from build123d import *

# Parameters (mm, degrees)
SKETCH1_W           = 30
SKETCH1_H           = 100
BOSS_EXTRUDE1_DEPTH = 10
SKETCH2_R           = 5
CUT_EXTRUDE1_DEPTH  = 10
SKETCH3_W           = 100
SKETCH3_H           = 40
BOSS_EXTRUDE2_DEPTH = 50
FILLET1_R           = 10


with BuildPart() as part:
    # Sketch1 → Boss-Extrude1 (new body)
    with BuildSketch(Plane(origin=(0, 0, 0), x_dir=(1, 0, 0), z_dir=(0, 1, 0))):
        Rectangle(SKETCH1_W, SKETCH1_H)
    extrude(amount=BOSS_EXTRUDE1_DEPTH)

    # Sketch2 → Cut-Extrude1 (cut)
    with BuildSketch(Plane(origin=(0, 10, 0), x_dir=(1, 0, 0), z_dir=(0, 1, 0))):
        with Locations(Location((0, -40, 0), (0, 0, 270))):
            Circle(SKETCH2_R)
    extrude(amount=-CUT_EXTRUDE1_DEPTH, mode=Mode.SUBTRACT)

    # Sketch3 → Boss-Extrude2 (add)
    with BuildSketch(Plane(origin=(0, 0, -50), x_dir=(-1, 0, 0), z_dir=(0, 0, -1))):
        with Locations((0, 5)):
            Rectangle(SKETCH3_W, SKETCH3_H)
    extrude(amount=-BOSS_EXTRUDE2_DEPTH)

    # Fillet1
    fillet1_edges = [part.edges().sort_by_distance(p)[0] for p in [
        (15, 5, 50),
        (-15, 5, 50),
    ]]
    fillet(fillet1_edges, radius=FILLET1_R)


solid = part.part
Model file for the job. Use its own axes, mm. A direction names the side the tool comes from. Give positions to 0.01 mm unless a question says otherwise; leave off trailing zeros. Loops run counter-clockwise (first coordinate to the right, second up) from the corner with the lowest first, then second, coordinate; pieces in that order, holes last.
Item 1: Drill centre lines: line 1 along X through (y, z) = (6, 40); line 2 along Z through (x, y) = (42, 18); line 3 along X through (y, z) = (2, 14). Where is each one in solid material? Low to high.
Check values:
line 1: x = -15 to -5, 5 to 15
line 2: z = -50 to 0
line 3: x = -15 to 15
Item 2: Slice it at A-A (x = 0). Write the cut outline in (y, z).
Check values:
outline: (-15, -50) - (25, -50) - (25, 0) - (10, 0) - (10, 35) - (0, 35) - (0, 0) - (-15, 0) - close; (0, 45) - (10, 45) - (10, 50) - (0, 50) - close
Item 3: Mould opens along X. For faces 6 (the face through (0, 5, 50)), 7 (the face through (15, 5, 20)), 8 (the face through (0, 5, 35)) say: +X half, -X half, draft (parallel to the pull), parting line (faces both ways), or undercut.
Check values:
face 6: draft
face 7: +X half
face 8: undercut
Item 4: Which spindle directions (+Z, -Z, +X, -X, +Y, -Y) get a long thin tool onto all of the face, cutting with end or side? Do faces 1 (the face through (50, 5, -25)), 2 (the face through (0, 10, 25)), 3 (the face through (0, 0, 25)), 4 (the face through (-15, 5, 20)), 5 (the face through (1, -15, -25)). Say none if no direction does.
Check values:
face 1: +Z, -Z, +X, +Y, -Y
face 2: +Z, +X, -X, +Y
face 3: +Z, +X, -X, -Y
face 4: +Z, -X, +Y, -Y
face 5: +Z, -Z, +X, -X, -Y
Item 5: Slice it at C-C (z = 20). Write the cut outline in (x, y).
Check values:
outline: (-15, 0) - (15, 0) - (15, 10) - (-15, 10) - close
Item 6: Slice it at B-B (y = -2). Write the cut outline in (x, z), plus the area to 3 significant figures.
Check values:
outline: (-50, -50) - (50, -50) - (50, 0) - (-50, 0) - close
area: 5,000 mm2
Item 7: Drop flat-ended pins along their axis: P1, Ø15, axis at x = 2, z = 25.5, coming from the -Y side; P2, Ø9, axis at x = 3, z = 19.5, coming from the +Y side; P3, Ø3, axis at y = 6.5, z = 20.5, coming from the +X side. Give the stop position or say it passes through.
Check values:
P1: stops at y = 0
P2: stops at y = 10
P3: stops at x = 15
